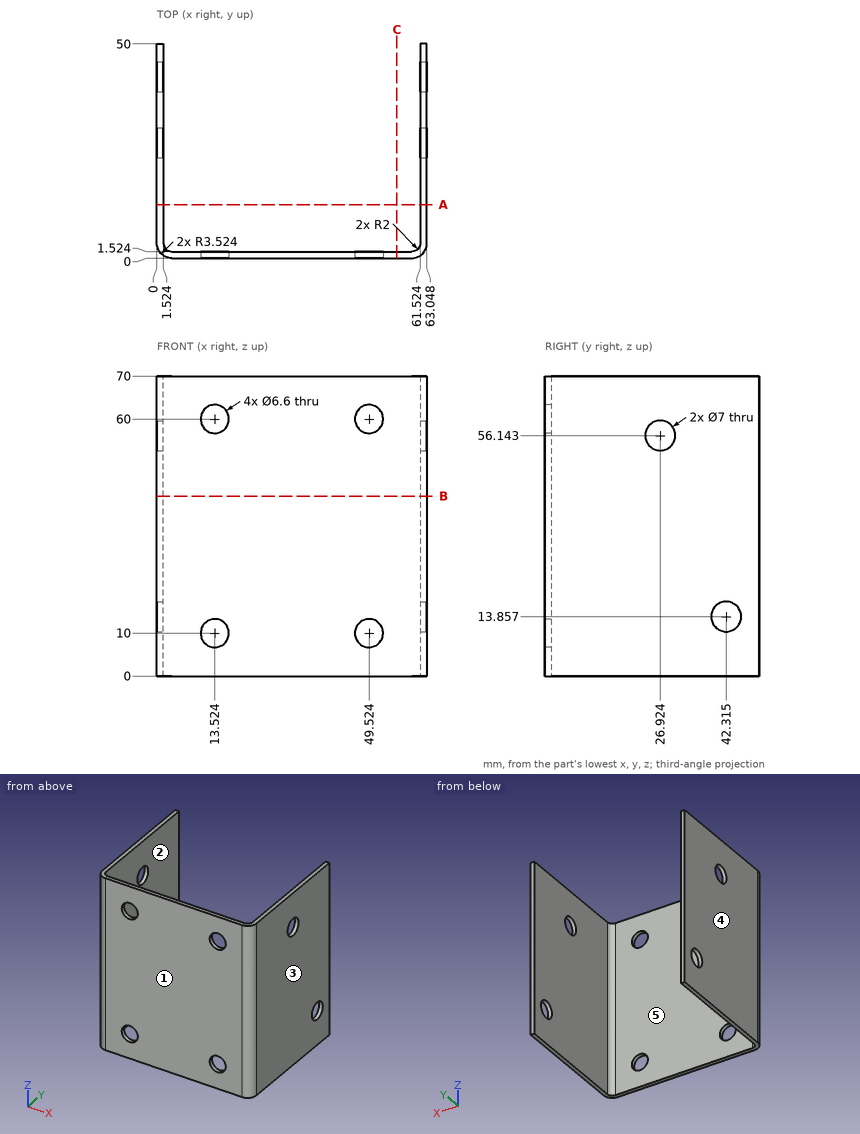
Source: three-view drawing plus pictorial views. Frame: mm from the lowest corner of the part. A direction names the side the tool comes from. Coordinates: 2 decimals unless noted, no trailing zeros. Loops run counter-clockwise (first coordinate to the right, second up) from the corner with the lowest first, then second, coordinate; pieces in that order, holes last. Notation, with made-up numbers: (-2.5, -29) - (7.5, -29) arc R23 cw to (7.5, -12) - close; hole circle Ø4 at (-36.5, -3.5). An arc over 180 degrees is marked (long way). Answer in a Markdown table with one row per item. Add a question column.
Item 1: Section query C-C on x = 56. Return the cut outline in (y, z), then the cut area to 3 significant figures.
Item 2: Mould query, pull axis X, two halves, no side actions, for the marked faces 1, 2 and 3. Classes: released by +X, released by -X, zero draft, split by the parting line, or undercut.
Item 3: Contact query for flat-ended pins moving along their axis: P1, Ø7.5, axis at x = 49.524, z = 10, coming from the +Y side; P2, Ø3, axis at x = 42.5, z = 43.5, coming from the -Y side; P3, Ø4, axis at y = 42.31, z = 13.86, coming from the +X side. Output: stop coordinate, or through.
Item 4: Section query B-B on z = 42. Return the cut outline in (x, y), then the cut area to 3 significant figures.
Item 5: Section query A-A on y = 12.5. Return the cut outline in (x, z), then the cut area to 3 significant figures.
Item 6: Access query for the marked faces 4 and 5. Directions: +Z, -Z, +X, -X, +Y, -Y. A direction counts if a zero-diameter tool reaches every point of the face in a straight line with its end or side. Return the directions, or none.
Item 7: Line query: line 1 along X through (y, z) = (6, 9); line 2 along Y through (x, z) = (59.5, 32.5). Output: solid intervals per line, ascending. Write a range as [from, to].
Recorded:
| question | item | result |
|---|---|---|
| 1 | outline | (0, 0) - (1.52, 0) - (1.52, 70) - (0, 70) - close |
| 1 | area | 107 mm^2 |
| 2 | face 1 | zero draft |
| 2 | face 2 | undercut |
| 2 | face 3 | released by +X |
| 3 | P1 | y = 1.52 |
| 3 | P2 | y = 0 |
| 3 | P3 | through |
| 4 | outline | (0, 3.52) arc R3.52 ccw to (3.52, 0) - (59.52, 0) arc R3.52 ccw to (63.05, 3.52) - (63.05, 50) - (61.52, 50) - (61.52, 3.52) arc R2 cw to (59.52, 1.52) - (3.52, 1.52) arc R2 cw to (1.52, 3.52) - (1.52, 50) - (0, 50) - close |
| 4 | area | 240 mm^2 |
| 5 | outline | (0, 0) - (1.52, 0) - (1.52, 70) - (0, 70) - close; (61.52, 0) - (63.05, 0) - (63.05, 70) - (61.52, 70) - close |
| 5 | area | 213 mm^2 |
| 6 | face 4 | +Z, -Z, -X, +Y, -Y |
| 6 | face 5 | +Z, -Z, +Y |
| 7 | line 1 | [0, 1.52], [61.52, 63.05] |
| 7 | line 2 | [0, 1.52] |
